The model under review builds one solid part; all positions refer to its coordinate system, in mm. Face numbers are marked on the shaded views. A direction names the side the tool comes from. Round coordinates to 2 decimals unless told otherwise and drop trailing zeros. Write each loop counter-clockwise with the first axis right and the second up, starting at its lowest first coordinate (ties: lowest second). Pieces come first, ordered by that corner, then holes.
Item 1: Add section D-D (x = 9.5). Give the boundary of the cut face in (y, z).
Item 2: To check wall thickness, follow L1, parallel to X at y = 5, z = 10.7; L2, parallel to X at y = 6, z = 5.5; L3, parallel to Y at x = 16, z = 10.05. State the ranges of each line that lie inside material, in increasing order.
Item 3: Clearance check with flat-ended pins moving along their axes: pin 1 Ø1.5 at (x, z) = (11, -2) entering from -Y; pin 2 Ø1.5 at (y, z) = (1, -2.5) entering from -X; pin 3 Ø4 at (y, z) = (6.5, -3) entering from +X; pin 4 Ø5 at (x, y) = (2, 6) entering from +Z. State where each tip first meets the part, or that it passes through.
Item 4: Add section B-B (y = 5). Give the boundary of the cut face in (x, z), plus the area to 3 significant figures.
Item 5: Draft analysis for pull direction X (two halves, no side actions). For the marked faces 1, 2, 3 and 4, state which applies: +X half, -X half, draft (parallel to the pull), parting line (faces both ways), or undercut.
Item 6: Add section C-C (y = 1.75). Give the boundary of the cut face in (x, z), plus the area to 3 significant figures.
Item 7: Add section A-A (z = -4.5). Give the boundary of the cut face in (x, y).
Item 8: Machinability: for the marked faces 5, 6, 7, 8 and 9, which of the approach directions +Z, -Z, +X, -X, +Y, -Y give a long, thin tool a straight path to every point of the face, cutting with its end or side? Answer none if there is none.
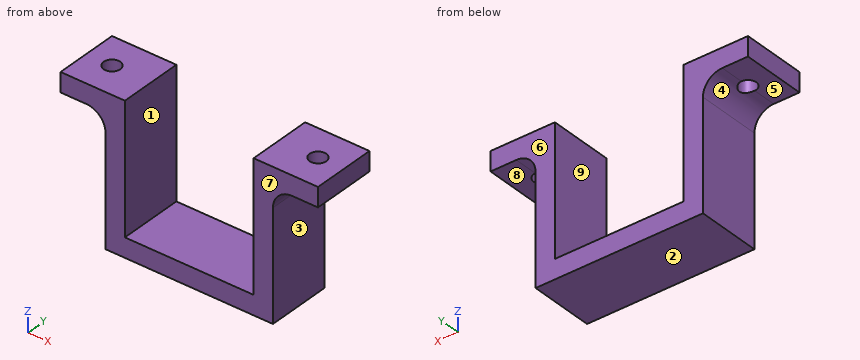
```python
from build123d import *

# Parameters (mm, degrees)
SKETCH_1_W          = 40
SKETCH_1_H          = 23
EXTRUDE_1_DEPTH     = 10
SKETCH_2_W          = 7
SKETCH_2_H          = 20
CUT_EXTRUDE_1_DEPTH = 10
SKETCH_3_W          = 20
SKETCH_3_H          = 20
CUT_EXTRUDE_2_DEPTH = 10
SKETCH_4_R          = 1.3
CUT_EXTRUDE_3_DEPTH = 10
FILLET_1_R          = 3
FILLET_2_R          = 3


with BuildPart() as part:
    # 草图1 → 凸台-拉伸1 (new body)
    with BuildSketch(Plane(origin=(0, 0, 0), x_dir=(1, 0, 0), z_dir=(0, 1, 0))):
        Rectangle(SKETCH_1_W, SKETCH_1_H)
    extrude(amount=EXTRUDE_1_DEPTH)

    # 草图2 → 切除-拉伸1 (cut)
    with BuildSketch(Plane(origin=(0, 10, 0), x_dir=(1, 0, 0), z_dir=(0, 1, 0))):
        with Locations((-16.5, 1.5)):
            Rectangle(SKETCH_2_W, SKETCH_2_H)
        with Locations((16.5, 1.5)):
            Rectangle(SKETCH_2_W, SKETCH_2_H)
    extrude(amount=-CUT_EXTRUDE_1_DEPTH, mode=Mode.SUBTRACT)

    # 草图3 → 切除-拉伸2 (cut)
    with BuildSketch(Plane(origin=(0, 10, 0), x_dir=(1, 0, 0), z_dir=(0, 1, 0))):
        with Locations((0, -1.5)):
            Rectangle(SKETCH_3_W, SKETCH_3_H)
    extrude(amount=-CUT_EXTRUDE_2_DEPTH, mode=Mode.SUBTRACT)

    # 草图4 → 切除-拉伸3 (cut)
    with BuildSketch(Plane(origin=(0, 0, 8.5), x_dir=(-1, 0, 0), z_dir=(0, 0, -1))):
        with Locations((16, 5)):
            Circle(SKETCH_4_R)
        with Locations((-16, 5)):
            Circle(SKETCH_4_R)
    extrude(amount=-CUT_EXTRUDE_3_DEPTH, mode=Mode.SUBTRACT)

    # 圆角1
    # the kernel refuses this fillet: 3 mm, written as the material it adds along each edge
    with BuildSketch(Plane(origin=(13, 10, 8.5), x_dir=(0, 0, -1), z_dir=(0, -1, 0))) as fillet_1_piece_1_section:
        with BuildLine():
            CenterArc((FILLET_1_R, FILLET_1_R), FILLET_1_R, 180, 90)
            Line((0, FILLET_1_R), (0, 0))
            Line((0, 0), (FILLET_1_R, 0))
        make_face()
    fillet_1_piece_1 = extrude(amount=10, mode=Mode.PRIVATE)
    fillet_1_piece_1 = fillet_1_piece_1 - Plane(origin=(16, 5, 7.810677701), x_dir=(-1, 0, 0), z_dir=(0, 0, -1)) * Cylinder(1.3, 32, mode=Mode.PRIVATE)
    add(fillet_1_piece_1)

    # 圆角2
    # the kernel refuses this fillet: 3 mm, written as the material it adds along each edge
    with BuildSketch(Plane(origin=(-13, 10, 8.5), x_dir=(0, 0, -1), z_dir=(0, -1, 0))) as fillet_2_piece_1_section:
        with BuildLine():
            CenterArc((FILLET_2_R, -FILLET_2_R), FILLET_2_R, 90, 90)
            Line((0, -FILLET_2_R), (0, 0))
            Line((0, 0), (FILLET_2_R, 0))
        make_face()
    fillet_2_piece_1 = extrude(amount=10, mode=Mode.PRIVATE)
    fillet_2_piece_1 = fillet_2_piece_1 - Plane(origin=(-16, 5, 7.810678225), x_dir=(-1, 0, 0), z_dir=(0, 0, -1)) * Cylinder(1.3, 32, mode=Mode.PRIVATE)
    add(fillet_2_piece_1)


solid = part.part
```
Numbers:
1. outline: (0, -11.5) - (10, -11.5) - (10, -8.5) - (0, -8.5) - close
2. L1: x = -20 to -17.3, -14.7 to -10, 10 to 14.7, 17.3 to 20
2. L2: x = -13 to -10, 10 to 13
2. L3: y = 0 to 3.7, 6.3 to 10
3. pin 1: stops at y = 0
3. pin 2: stops at x = -13
3. pin 3: stops at x = 13
3. pin 4: stops at z = -8.5
4. outline: (-20, 8.5) - (-17.3, 8.5) - (-17.3, 11.5) - (-20, 11.5) - close; (-14.7, 8.2) arc R3 cw to (-13, 5.5) - (-13, -11.5) - (13, -11.5) - (13, 5.5) arc R3 cw to (14.7, 8.2) - (14.7, 11.5) - (10, 11.5) - (10, -8.5) - (-10, -8.5) - (-10, 11.5) - (-14.7, 11.5) - close; (17.3, 8.5) - (20, 8.5) - (20, 11.5) - (17.3, 11.5) - close
4. area: 228 mm2
5. face 1: undercut
5. face 2: draft
5. face 3: +X half
5. face 4: -X half
6. outline: (-20, 8.5) - (-16, 8.5) arc R3 cw to (-13, 5.5) - (-13, -11.5) - (13, -11.5) - (13, 5.5) arc R3 cw to (16, 8.5) - (20, 8.5) - (20, 11.5) - (10, 11.5) - (10, -8.5) - (-10, -8.5) - (-10, 11.5) - (-20, 11.5) - close
6. area: 244 mm2
7. outline: (-13, 0) - (-10, 0) - (-10, 10) - (-13, 10) - close; (10, 0) - (13, 0) - (13, 10) - (10, 10) - close
8. face 5: -Z, -X, +Y, -Y
8. face 6: +Z, -Z, +X, -X, +Y
8. face 7: +Z, -Z, +X, -X, -Y
8. face 8: -Z, +X, +Y, -Y
8. face 9: +Z, +Y, -Y
